from build123d import *

# Parameters (mm, degrees)
EXTRUDE_1_DEPTH     = 60
SKETCH_3_W          = 15
SKETCH_3_H          = 8
CUT_EXTRUDE_1_DEPTH = 50


with BuildPart() as part:
    # 草图1 → 凸台-拉伸1 (new body)
    with BuildSketch(Plane.XY):
        Polygon((-37.017562776, 4), (-27.017562776, 4), (-27.017562776, 2), (-22.017562776, 2), (-22.017562776, 0), (-17.017562776, 0), (-17.017562776, -2), (-12.017562776, -2), (-12.017562776, -4), (-7.017562776, -4), (-7.017562776, -6), (-7.017562776, -17.776315497), (-57.017562776, -17.776315497), (-57.017562776, -6), (-57.017562776, -4), (-52.017562776, -4), (-52.017562776, -2), (-47.017562776, -2), (-47.017562776, 0), (-42.017562776, 0), (-42.017562776, 2), (-37.017562776, 2), align=None)
    extrude(amount=EXTRUDE_1_DEPTH)

    # 草图3 → 切除-拉伸1 (cut)
    with BuildSketch(Plane(origin=(-7.017562776, 0, 0), x_dir=(0, 0, -1), z_dir=(1, 0, 0))):
        with Locations((-52.5, 0)):
            Rectangle(SKETCH_3_W, SKETCH_3_H)
    extrude(amount=-CUT_EXTRUDE_1_DEPTH, mode=Mode.SUBTRACT)


solid = part.part
Work out the finished part from the listing and answer in its coordinate system (mm). A direction names the side the tool comes from. Coordinates: 2 decimals unless noted, no trailing zeros. Write each loop counter-clockwise with the first axis right and the second up, starting at its lowest first coordinate (ties: lowest second). Pieces come first, ordered by that corner, then holes. Notation, with made-up numbers: M 70,59 L 111,59 A22 ccw 111,81 Z; hole C -38,75 d11. An arc over 180 degrees is marked long. Write item = value, one per line.
1. Straight lines are drawn through the part: line 1 (Y direction, x = -46.5, z = 3); line 2 (Y direction, x = -50, z = 15); line 3 (X direction, y = -1, z = 24). For each, find the intervals that lie inside material, in ascending order. Write a range as from..to.
Solution:
line_1 = -17.78..0
line_2 = -17.78..-2
line_3 = -47.02..-17.02
2. The part is cut by section C-C (y = -1). Determine the outline of the cut face in (x, z), then the cut area to 3 significant figures.
Solution:
outline = M -47.02,0 L -17.02,0 L -17.02,45 L -47.02,45 Z
area = 1,350 mm2
3. The part is cut by section A-A (x = -23.5). Determine the outline of the cut face in (y, z), then the cut area to 3 significant figures.
Solution:
outline = M -17.78,0 L 2,0 L 2,45 L -4,45 L -4,60 L -17.78,60 Z
area = 1,100 mm2
4. The part is cut by section B-B (z = 39.5). Determine the outline of the cut face in (x, y).
Solution:
outline = M -57.02,-17.78 L -7.02,-17.78 L -7.02,-4 L -12.02,-4 L -12.02,-2 L -17.02,-2 L -17.02,0 L -22.02,0 L -22.02,2 L -27.02,2 L -27.02,4 L -37.02,4 L -37.02,2 L -42.02,2 L -42.02,0 L -47.02,0 L -47.02,-2 L -52.02,-2 L -52.02,-4 L -57.02,-4 Z
5. Flat-ended cylindrical pins translate along their axes: pin 1 (5.5 mm diameter, centred on x = -49, z = 24, fed in from +Y); pin 2 (5.5 mm diameter, centred on x = -20, z = 23, fed in from +Y); pin 3 (1.6 mm diameter, centred on y = -1, z = 16.5, fed in from -X). Find the tip coordinate at first contact, or state that the pin passes through.
Solution:
pin_1 = 0
pin_2 = 2
pin_3 = -47.02
6. For faces 1 (the face through (-40, 2, 22)), 2 (the face through (-32, -1, 45)), 3 (the face through (-12.018, -3, 22)), determine the directions among +Z, -Z, +X, -X, +Y, -Y from which every point of the face is accessible in a straight line to the end or side of a thin tool.
Solution:
face_1 = +Z, -Z, -X, +Y
face_2 = +Z, +X, -X, +Y
face_3 = +Z, -Z, +X, +Y
7. The part is cut by section D-D (x = -45.5). Determine the outline of the cut face in (y, z).
Solution:
outline = M -17.78,0 L 0,0 L 0,45 L -4,45 L -4,60 L -17.78,60 Z
